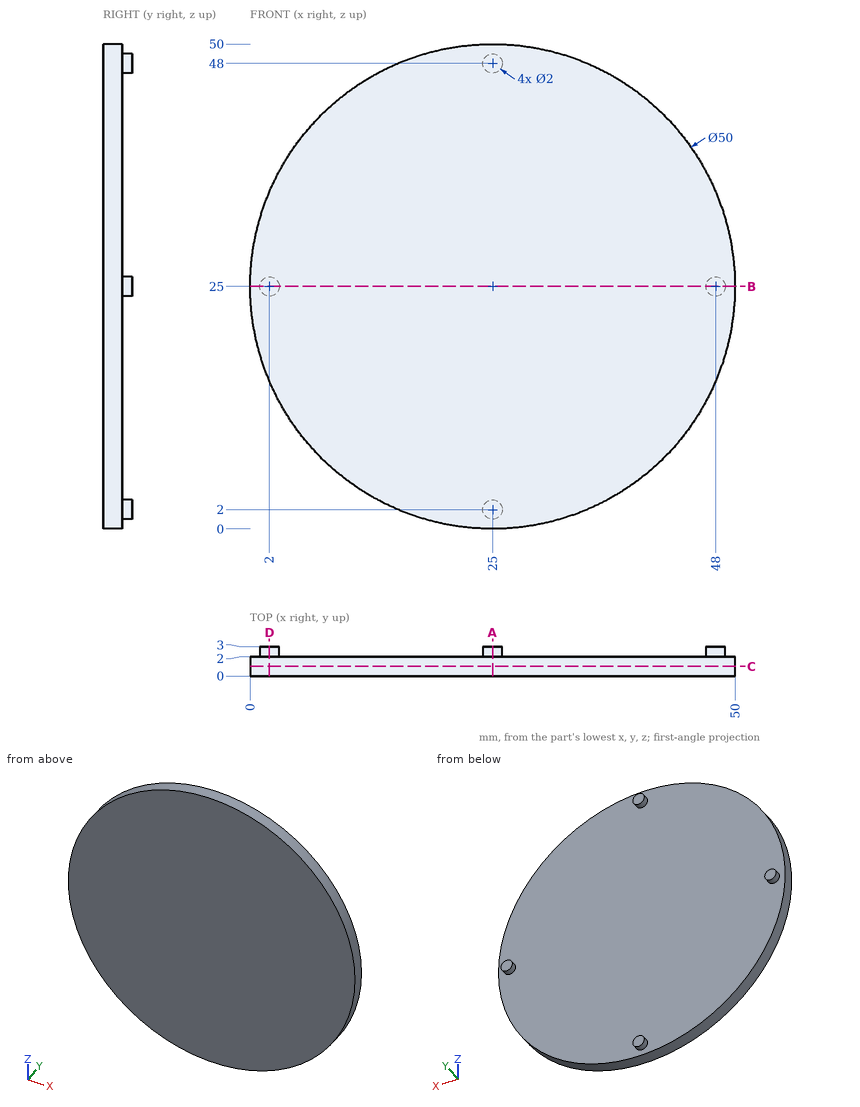
The figure shows three views and two pictorial views of one solid part (mm, origin at its lowest corner). Answer the questions. Coordinates: 2 decimals unless noted, no trailing zeros. Loops run counter-clockwise (first coordinate to the right, second up) from the corner with the lowest first, then second, coordinate; pieces in that order, holes last.
(1) Flat-ended cylindrical pins translate along their axes: pin 1 Ø3 at (x, z) = (37, 26) entering from +Y; pin 2 Ø1 at (x, y) = (29, 2) entering from +Z. Find the tip coordinate at first contact, or state that the pin passes through.
Solution:
pin 1: stops at y = 2
pin 2: stops at z = 49.75
(2) The part is cut by section A-A (x = 25). Determine the outline of the cut face in (y, z), and give its area (3 significant figures).
Solution:
outline: (0, 0) - (2, 0) - (2, 1) - (3, 1) - (3, 3) - (2, 3) - (2, 47) - (3, 47) - (3, 49) - (2, 49) - (2, 50) - (0, 50) - close
area: 104 mm2
(3) The part is cut by section D-D (x = 2). Determine the outline of the cut face in (y, z), and give its area (3 significant figures).
Solution:
outline: (0, 15.2) - (2, 15.2) - (2, 24) - (3, 24) - (3, 26) - (2, 26) - (2, 34.8) - (0, 34.8) - close
area: 41.2 mm2
(4) The part is cut by section C-C (y = 1). Determine the outline of the cut face in (x, z), and give its area (3 significant figures).
Solution:
outline: circle Ø50 at (25, 25)
area: 1,960 mm2
(5) Consider line 1 along Y through (x, z) = (9, 12); line 2 along X through (y, z) = (0.2, 32); line 3 along Z through (x, y) = (24.5, 0.1) (3 decimals). Determine where each line is inside the solid, lowest interval first.
Solution:
line 1: y = 0 to 2
line 2: x = 1 to 49
line 3: z = 0.005 to 49.995
(6) The part is cut by section B-B (z = 25). Determine the outline of the cut face in (x, y).
Solution:
outline: (0, 0) - (50, 0) - (50, 2) - (49, 2) - (49, 3) - (47, 3) - (47, 2) - (3, 2) - (3, 3) - (1, 3) - (1, 2) - (0, 2) - close
